```python
from build123d import *

# Parameters (mm, degrees)
BOSS_EXTRUDE1_DEPTH = 5
BOSS_EXTRUDE2_START = 5
BOSS_EXTRUDE2_DEPTH = 24
SKETCH7_R           = 1.1
CUT_EXTRUDE1_DEPTH  = 71.543483188


with BuildPart() as part:
    # Sketch1 → Boss-Extrude1 (new body)
    with BuildSketch(Plane.XY):
        with BuildLine():
            Line((-36.5125, 46.0375), (36.5125, 46.0375))
            ThreePointArc((36.5125, 46.0375), (47.737820151, 41.387820151), (52.3875, 30.1625))
            Line((52.3875, 30.1625), (52.3875, -30.1625))
            ThreePointArc((52.3875, -30.1625), (47.737820151, -41.387820151), (36.5125, -46.0375))
            Line((36.5125, -46.0375), (-36.5125, -46.0375))
            ThreePointArc((-36.5125, -46.0375), (-47.737820151, -41.387820151), (-52.3875, -30.1625))
            Line((-52.3875, -30.1625), (-52.3875, 30.1625))
            ThreePointArc((-52.3875, 30.1625), (-47.737820151, 41.387820151), (-36.5125, 46.0375))
        make_face()
    extrude(amount=BOSS_EXTRUDE1_DEPTH)

    # Sketch5 → Boss-Extrude2 (add)
    with BuildSketch(Plane(origin=(0, 0, 0), x_dir=(1, 0, 0), z_dir=(0, 1, 0)).offset(BOSS_EXTRUDE2_START)):
        Polygon((5, -5), (35, -10.233130218), (35, -5), align=None)
    extrude(amount=BOSS_EXTRUDE2_DEPTH)

    # Sketch7 → Cut-Extrude1 (cut, through all)
    with BuildSketch(Plane(origin=(-0.698782941, 0, 4.005917559), x_dir=(0.985124383035979, 0, 0.17184280592443155), z_dir=(-0.17184280592443155, 0, 0.985124383035979))):
        with Locations((10.511339581, 23)):
            Circle(SKETCH7_R)
        with Locations(Location((31.511339581, 23, 0), (0, 0, 180))):
            Circle(SKETCH7_R)
        with Locations((31.511339581, 10.5)):
            Circle(SKETCH7_R)
        with Locations(Location((10.511339581, 10.5, 0), (0, 0, 180))):
            Circle(SKETCH7_R)
        with BuildLine():
            Line((29.411339581, 27), (12.611339581, 27))
            Line((12.611339581, 27), (12.611339581, 23))
            ThreePointArc((12.611339581, 23), (11.996263821, 21.51507576), (10.511339581, 20.9))
            Line((10.511339581, 20.9), (8.511339581, 20.9))
            Line((8.511339581, 20.9), (8.511339581, 12.6))
            Line((8.511339581, 12.6), (10.511339581, 12.6))
            ThreePointArc((10.511339581, 12.6), (11.996263821, 11.98492424), (12.611339581, 10.5))
            Line((12.611339581, 10.5), (12.611339581, 6.5))
            Line((12.611339581, 6.5), (29.411339581, 6.5))
            Line((29.411339581, 6.5), (29.411339581, 10.5))
            ThreePointArc((29.411339581, 10.5), (30.02641534, 11.98492424), (31.511339581, 12.6))
            Line((31.511339581, 12.6), (33.511339581, 12.6))
            Line((33.511339581, 12.6), (33.511339581, 20.9))
            Line((33.511339581, 20.9), (31.511339581, 20.9))
            ThreePointArc((31.511339581, 20.9), (30.02641534, 21.51507576), (29.411339581, 23))
            Line((29.411339581, 23), (29.411339581, 27))
        make_face()
    extrude(amount=-CUT_EXTRUDE1_DEPTH, mode=Mode.SUBTRACT)


solid = part.part
```
Work out the finished part from the listing and answer in its coordinate system (mm). A direction names the side the tool comes from. Round coordinates to 2 decimals unless told otherwise and drop trailing zeros. Loops run counter-clockwise (first coordinate to the right, second up) from the corner with the lowest first, then second, coordinate; pieces in that order, holes last. Notation, with made-up numbers: (-37.5, -26.5) -> (-31.5, -26.5) arc R29 ccw to (-31.5, 6.5) -> close; hole circle Ø2 at (70.5, -6). An arc over 180 degrees is marked (long way). Write each question's results on one line, items separated by ' | '. Start each with the question number.
1. A tool of negligible diameter and unlimited length cuts with its end or side. For faces 4 (the face through (26, 29, 6)), 5 (the face through (32, 20.9, 5)), 6 (the face through (9, 20.9, 3)), from which of +Z, -Z, +X, -X, +Y, -Y can it reach the whole face along a straight path? Write none if from no direction.
2. Find the intervals of material crossed by probe 1 along Z at (x, y) = (10.5, -34); probe 2 along Y at (x, z) = (12, 2); probe 3 along X at (y, z) = (8.5, 4.75), in increasing order. Write a range as from..to.
3. Section A-A (y = 19.5) is taken. Determine the outline of the cut face in (x, z).
4. For a pull along Y with two mould halves and no side action, classify faces 1 (the face through (20, 6.5, 4)), 2 (the face through (47.861, -41.264, 2.465)), 3 (the face through (35, 17, 8)) as +Y half, -Y half, draft (parallel to the pull), parting line (faces both ways), or undercut.
5. Section D-D (y = -25) is taken. Determine the outline of the cut face in (x, z).
6. Given pin 1 Ø1.6 at (x, z) = (13.5, 8.5) entering from -Y; pin 2 Ø4 at (x, y) = (-0.5, 18.5) entering from +Z; pin 3 Ø1.6 at (x, z) = (20, 8) entering from +Y; pin 4 Ø1.8 at (x, z) = (32.5, 6) entering from -Y, each flat-ended and moving along its own axis, determine where each tip first touches the part or whether it passes through.
7. Section B-B (x = 14) is taken. Determine the outline of the cut face in (y, z).
8. Section C-C (z = 7.5) is taken. State how many separate pieces and enclosed holes the cut face has, plus the area to 3 significant figures.
Evaluation:
1) face 4: +Z, +X, -X, +Y | face 5: -Z | face 6: +Z
2) probe 1: z = 0..5 | probe 2: y = -46.04..11.79, 21.71..46.04 | probe 3: x = -52.39..11.97, 29.03..52.39
3) outline: (-52.39, 0) -> (8.64, 0) -> (7.69, 5.47) -> (5, 5) -> (-52.39, 5) -> close; (32.31, 9.76) -> (34.02, 0) -> (52.39, 0) -> (52.39, 5) -> (35, 5) -> (35, 10.23) -> close
4) face 1: undercut | face 2: -Y half | face 3: draft
5) outline: (-52.39, 0) -> (52.39, 0) -> (52.39, 5) -> (-52.39, 5) -> close
6) pin 1: passes through | pin 2: stops at z = 5 | pin 3: stops at y = 29 | pin 4: stops at y = 5
7) outline: (-46.04, 0) -> (6.5, 0) -> (6.5, 6.57) -> (5, 6.57) -> (5, 5) -> (-46.04, 5) -> close; (27, 0) -> (46.04, 0) -> (46.04, 5) -> (29, 5) -> (29, 6.57) -> (27, 6.57) -> close
8) separate pieces: 1 | enclosed holes: 2 | area: 143 mm2
